The drawing under review shows one solid part. Ordinate dimensions are in mm from its lowest x, y, z. A direction names the side the tool comes from. Coordinates: 2 decimals unless noted, no trailing zeros. Loops run counter-clockwise (first coordinate to the right, second up) from the corner with the lowest first, then second, coordinate; pieces in that order, holes last. Notation, with made-up numbers: (-14.5, 74.5) - (-4.5, 74.5) arc R12 ccw to (-4.5, 82.5) - close; hole circle Ø6 at (80.25, 8). An arc over 180 degrees is marked (long way). Answer as a JSON object with one key per item and string values. Group by question number.
Item 1: Clearance check with flat-ended pins moving along their axes: pin 1 (1.6 mm diameter, centred on x = 25.36, z = 5.16, fed in from -Y); pin 2 (1 mm diameter, centred on y = 2.5, z = 20, fed in from -X); pin 3 (2 mm diameter, centred on x = 21.5, y = 2, fed in from -Z); pin 4 (1.3 mm diameter, centred on x = 25, z = 6, fed in from +Y). State where each tip first meets the part, or that it passes through.
Item 2: We need section A-A (x = 25.36). Give the boundary of the cut face in (y, z), then the cut area to 3 significant figures.
Item 3: We need section C-C (y = 1.5). Give the boundary of the cut face in (x, z).
Item 4: To check wall thickness, follow line 1 (X direction, y = 1.25, z = 20.16); line 2 (X direction, y = 3.25, z = 28.5); line 3 (Z direction, x = 34, y = 0.45). State the ranges of each line that lie inside material, in increasing order.
Item 5: Tool access review of the marked faces 1, 2 and 3: name each direction out of +Z, -Z, +X, -X, +Y, -Y from which nothing blocks a thin tool from reaching the whole face with its end or side.
Item 6: We need section D-D (z = 5). Give the boundary of the cut face in (x, y).
Item 7: We need section B-B (z = 20.16). Give the boundary of the cut face in (x, y), then the cut area to 3 significant figures.
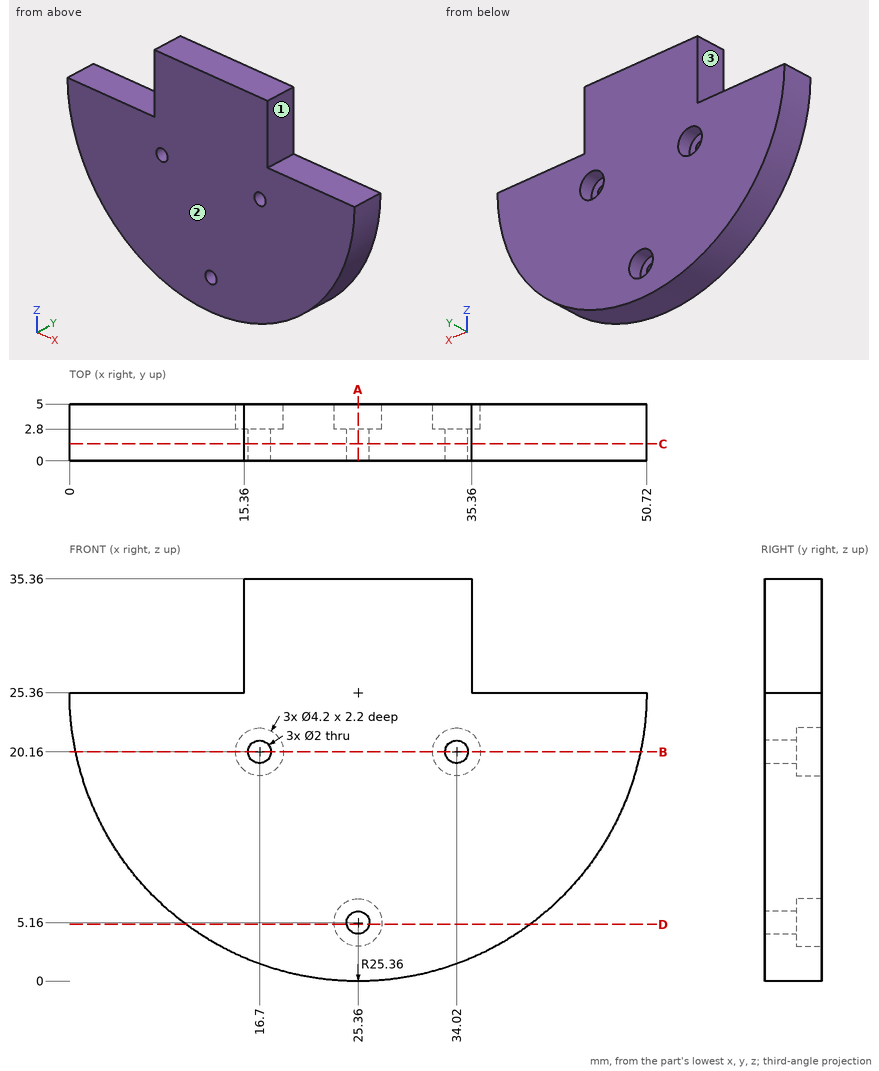
Check sheet entries:
{
 "1": {"pin 1": "passes through", "pin 2": "stops at x = 0.47", "pin 3": "stops at z = 0.16", "pin 4": "stops at y = 2.8"},
 "2": {"outline": "(0, 0) - (5, 0) - (5, 3.06) - (2.8, 3.06) - (2.8, 4.16) - (0, 4.16) - close; (0, 6.16) - (2.8, 6.16) - (2.8, 7.26) - (5, 7.26) - (5, 35.36) - (0, 35.36) - close", "area": "162 mm2"},
 "3": {"outline": "(0, 25.36) arc R25.36 ccw to (50.72, 25.36) - (35.36, 25.36) - (35.36, 35.36) - (15.36, 35.36) - (15.36, 25.36) - close; hole circle Ø2 at (16.7, 20.16); hole circle Ø2 at (25.36, 5.16); hole circle Ø2 at (34.02, 20.16)"},
 "4": {"line 1": "x = 0.54 to 15.7, 17.7 to 33.02, 35.02 to 50.18", "line 2": "x = 15.36 to 35.36", "line 3": "z = 1.52 to 19.16, 21.16 to 35.36"},
 "5": {"face 1": "+Z, +X, +Y, -Y", "face 2": "+Z, -Z, +X, -X, -Y", "face 3": "+Z, -X, +Y, -Y"},
 "6": {"outline": "(10.24, 0) - (24.37, 0) - (24.37, 2.8) - (23.27, 2.8) - (23.27, 5) - (10.24, 5) - close; (26.35, 0) - (40.48, 0) - (40.48, 5) - (27.45, 5) - (27.45, 2.8) - (26.35, 2.8) - close"},
 "7": {"outline": "(0.54, 0) - (15.7, 0) - (15.7, 2.8) - (14.6, 2.8) - (14.6, 5) - (0.54, 5) - close; (17.7, 0) - (33.02, 0) - (33.02, 2.8) - (31.92, 2.8) - (31.92, 5) - (18.8, 5) - (18.8, 2.8) - (17.7, 2.8) - close; (35.02, 0) - (50.18, 0) - (50.18, 5) - (36.12, 5) - (36.12, 2.8) - (35.02, 2.8) - close", "area": "219 mm2"}
}
